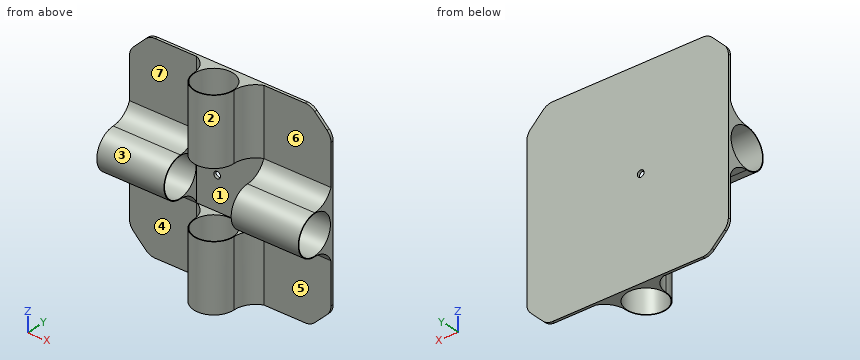
Autodesk Inventor part; units mm, degrees
ref_plane "YZ Plane" through (0, 0, 0) normal (1, 0, 0) x (0, 1, 0)
ref_plane "XZ Plane" through (0, 0, 0) normal (0, 1, 0) x (-1, 0, 0)
ref_plane "XY Plane" through (0, 0, 0) normal (0, 0, 1) x (1, 0, 0)
sketch "Sketch1" plane through (0, 0, 0) normal (0, 1, 0) x (-1, 0, 0)
  line L0 (75, 0) -> (75, 75)
  line L1 (75, 75) -> (-75, 75)
  line L2 (-75, 75) -> (-75, -75)
  line L3 (-75, -75) -> (75, -75)
  line L4 (75, -75) -> (75, 0)
  point P0 (0, 0)
  dimension "d0" = 75
  dimension "d1" = 75
  dimension "d2" = 150
  dimension "d3" = 150
extrude "Extrusion1" add sketch "Sketch1" along normal blind 2
sketch "Sketch2" plane through (0, 0, 0) normal (0, -1, 0) x (1, 0, 0)
  line L0 (75, 75) -> (75, 0)
  line L1 (75, 75) -> (75, -75)
  line L2 (75, 0) -> (75, 15)
  line L3 (75, 0) -> (75, -15)
  point P0 (0, 0)
  dimension "d6" = 15
  dimension "d7" = 15
sketch "Sketch3" plane through (75, 0, 75) normal (1, 0, 0) x (0, 0, -1)
  line L0 (75, 0) -> (90, 0)
  line L1 (150, 0) -> (0, 0)
  line L2 (75, 0) -> (60, 0)
  circle A0 centre (75.0005, -15) radius 15
  circle A1 centre (75.0005, -15) radius 14.5
  line L3 (60, 0) -> (50, 0)
  arc A2 (60.0008, -14.9109) -> (50, 0) centre (44.0261, -14.8159) ccw
  arc A3 (100.001, 0) -> (90.0002, -14.9109) centre (105.9749, -14.8159) ccw
  line L4 (50, 0) -> (75, 0)
  line L5 (100.001, 0) -> (75, 0)
  dimension "d8" = 15
  dimension "d10" = 15
  dimension "d13" = 10
extrude "Extrusion2" add sketch "Sketch3" against normal blind 50
pattern_circular "Circular Pattern1" count 4 over 360 about axis through (0, -10, 0) along (0, 1, 0) of "Extrusion2"
sketch "Sketch4" plane through (0, 0, 0) normal (0, 1, 0) x (-1, 0, 0)
  line L0 (-75, 75) -> (-75, 60)
  line L1 (-75, 75) -> (-75, -75)
  line L2 (-75, 75) -> (-60, 75)
  line L3 (-25.001, 75) -> (-75, 75)
  line L4 (-60, 75) -> (-75, 60)
  line L5 (-75, 60) -> (-60, 75)
  point P0 (0, 0)
  dimension "d19" = 15
  dimension "d20" = 15
extrude "Extrusion3" cut sketch "Sketch4" along normal blind 50
sketch "Sketch5" plane through (0, 2, 0) normal (0, 1, 0) x (1, 0, 0)
  line L0 (75, 75) -> (75, 60)
  line L1 (75, -60) -> (75, 75)
  line L2 (75, 60) -> (-75, 60)
  line L3 (75, 75) -> (-75, 75)
  line L4 (-75, 75) -> (-60, 75)
  line L5 (-60, 75) -> (-60, -75)
  line L6 (-75, -75) -> (-25, -75)
  line L7 (-75, -75) -> (-75, -60)
  line L8 (-75, 75) -> (-75, -75)
  line L9 (-75, -60) -> (-60, -60)
  line L10 (75, 75) -> (60, 75)
  line L11 (60, 75) -> (60, 60)
  line L12 (-60, -75) -> (-75, -60)
  line L13 (-60, 75) -> (-75, 60)
  line L14 (75, 60) -> (60, 75)
  point P0 (0, 0)
  dimension "d23" = 15
  dimension "d24" = 15
  dimension "d25" = 15
extrude "Extrusion4" cut sketch "Sketch5" against normal blind 50 contours L12 L6 L7
sketch "Sketch6" plane through (0, 2, 0) normal (0, 1, 0) x (1, 0, 0)
  line L0 (75, 75) -> (75, 60)
  line L1 (75, -60) -> (75, 75)
  line L2 (75, 60) -> (60, 60)
  line L3 (60, 60) -> (60, 75)
  line L4 (75, 75) -> (-75, 75)
  line L5 (75, 60) -> (60, 75)
  point P0 (0, 0)
  dimension "d28" = 15
  dimension "d29" = 15
extrude "Extrusion5" cut sketch "Sketch6" against normal blind 50 contours L0 L5 L4
sketch "Sketch7" plane through (0, 2, 0) normal (0, 1, 0) x (1, 0, 0)
  point P0 (0, 0)
sketch "Sketch8" plane through (0, 2, 0) normal (0, 1, 0) x (1, 0, 0)
  line L0 (-75, 75) -> (-60, 75)
  line L1 (60, 75) -> (-75, 75)
  line L2 (-60, 75) -> (-60, 60)
  line L3 (-60, 60) -> (-75, 60)
  line L4 (-75, 75) -> (-75, -60)
  line L5 (-60, 75) -> (-75, 60)
  point P0 (0, 0)
  dimension "d32" = 15
  dimension "d33" = 15
extrude "Extrusion6" cut sketch "Sketch8" against normal blind 50 contours L0 L5 L4
fillet "Fillet1" radius 10 2 edges at (60, 1, -75) (75, 1, -60)
pattern_circular "Circular Pattern2" count 4 over 360 about axis through (0, -10, 0) along (0, 1, 0) of "Fillet1"
sketch "Sketch9" plane through (0, 2, 0) normal (0, 1, 0) x (1, 0, 0)
  circle A0 centre (-9.7626, 0) radius 2.5
  point P0 (0, 0)
  dimension "d40" = 5
extrude "Extrusion7" cut sketch "Sketch9" against normal blind 5
equation "\"BendRadius\" = Thickness"
equation "\"BendReliefWidth\" = Thickness"
equation "\"BendReliefDepth\" = 0.5 * Thickness"
equation "\"CornerReliefSize\" = 4 * Thickness"
equation "\"MinimumRemnant\" = 2 * Thickness"
equation "\"TransitionRadius\" = BendRadius"
equation "\"JacobiRadiusSize\" = BendRadius"
equation "\"GapSize\" = Thickness"
properties part number "sqaureBase"
Work out the finished part from the listing and answer in its coordinate system (mm). Face numbers are marked on the shaded views. A direction names the side the tool comes from. Give positions to 0.01 mm unless a question says otherwise; leave off trailing zeros. Order: outer loops, then holes, each group sorted by start corner. A loop starts at its lowest first (then second) coordinate and runs counter-clockwise, first axis right, second up. Notation, with made-up numbers: (68, -14.5) - (126, -14.5) arc R26 cw to (126, 17.5) - close; hole circle Ø3 at (44, 5). An arc over 180 degrees is marked (long way). Answer as CSV lines item,"result". Start each with the question number.
Q1. The part is cut by section A-A (y = -4.5). Give the number of separate pieces and of enclosed holes in the cut face, then the cut area to 3 significant figures.
Q2. The part is cut by section C-C (x = -3.5). Write down the section's boundary in (y, z).
Q3. The part is cut by section B-B (z = 0). Write down the section's boundary in (x, y).
Q4. Find the intervals of material crossed by L1, parallel to X at y = 1.5, z = 0; L2, parallel to Y at x = -20, z = -19; L3, parallel to Y at x = 60, z = -12, in increasing order. Write a range as [from, to].
Q5. The part is cut by section D-D (x = 43). Write down the section's boundary in (y, z) (1 decimal), then the cut area to 3 significant figures.
Q6. For the marked faces 4, 5, 6 and 7, determine the directions among +Z, -Z, +X, -X, +Y, -Y from which every point of the face is accessible in a straight line to the end or side of a thin tool.
Q7. The mould has two halves that part along X. Classify the marked faces 1, 2 and 3: +X half, -X half, draft (parallel to the pull), parting line (faces both ways), or undercut.
Q8. Given pin 1 Ø15 at (y, z) = (-16, 10) entering from -X; pin 2 Ø1 at (x, z) = (-13.5, 35) entering from -Y; pin 3 Ø25 at (x, z) = (40, -39) entering from -Y; pin 4 Ø5 at (x, z) = (-44, 15) entering from -Y, each flat-ended and moving along its own axis, determine where each tip first touches the part or whether it passes through.
Check result:
1,separate pieces,"8"
1,enclosed holes,"0"
1,area,"3,510 mm²"
2,outline,"(-29.59, -75) - (-29.07, -75) - (-29.07, -25) - (-29.59, -25) - close; (-29.59, 25) - (-29.07, 25) - (-29.07, 75) - (-29.59, 75) - close; (-0.93, -75) - (2, -75) - (2, 75) - (-0.93, 75) - (-0.93, 25) - (0, 25) - (0, -25) - (-0.93, -25) - close"
3,outline,"(-75, -30) - (-25, -30) - (-25, -29.5) - (-75, -29.5) - close; (-75, -0.5) - (-25, -0.5) - (-25, 0) - (-12.26, 0) - (-12.26, 2) - (-75, 2) - close; (-7.26, 0) - (25, 0) - (25, -0.5) - (75, -0.5) - (75, 2) - (-7.26, 2) - close; (25, -30) - (75, -30) - (75, -29.5) - (25, -29.5) - close"
4,L1,"x = [-75, -12.26], [-7.26, 75]"
4,L2,"y = [0, 2]"
4,L3,"y = [-24, -23.14], [-6.86, 2]"
5,outline,"(-14.9, -15) arc R16 cw to (0, -25) - (0, -75) - (2, -75) - (2, 75) - (0, 75) - (0, 25) arc R16 cw to (-14.9, 15) arc R15 ccw (long way) to start; hole circle Ø29 at (-15, 0)"
5,area,"525 mm²"
6,face 4,"-Z, -X, -Y"
6,face 5,"-Z, +X, -Y"
6,face 6,"+Z, +X, -Y"
6,face 7,"+Z, -X, -Y"
7,face 1,"undercut"
7,face 2,"parting line"
7,face 3,"draft"
8,pin 1,"stops at x = -75"
8,pin 2,"stops at y = -22.48"
8,pin 3,"stops at y = 0"
8,pin 4,"stops at y = -23.29"
